from build123d import *

# Parameters (mm, degrees)
F1_DEPTH  = 495.3
F3_DEPTH  = 101.6
F4_R      = 63.5
F5_DEPTH  = 101.6
F7_DEPTH  = 127
F9_DEPTH  = 127
F11_DEPTH = 127
F13_DEPTH = 127


with BuildPart() as f1:
    # F0 (on Front) → F1 (new body)
    with BuildSketch(Plane.XZ):
        Polygon((635, -24.13), (635, 24.13), (-635, 24.13), (-635, 14.952256), (-635, -24.13), align=None)
        with BuildLine():
            Line((-635, -24.13), (-635, 14.952256))
            ThreePointArc((-635, 14.952256), (-763.72663, 119.691568), (-687.35112, 267.026731))
            Line((-687.35112, 267.026731), (-272.463288, 681.914564))
            Line((-272.463288, 681.914564), (-306.588261, 716.039537))
            Line((-306.588261, 716.039537), (-755.601067, 267.026731))
            ThreePointArc((-755.601067, 267.026731), (-792.572888, 81.156837), (-635, -24.13))
        make_face()
    extrude(amount=F1_DEPTH)

    # F2 (on face) → F3 (cut)
    with BuildSketch(Plane(origin=(-511.313899, 0, 511.313899), x_dir=(0, -1, 0), z_dir=(-0.707107, 0, 0.707107))):
        with BuildLine():
            ThreePointArc((152.4, 99.025774), (141.240768, 125.966543), (114.3, 137.125774))
            ThreePointArc((114.3, 137.125774), (87.359232, 72.085006), (152.4, 99.025774))
        make_face()
        with BuildLine():
            ThreePointArc((419.1, 99.025774), (407.940768, 125.966543), (381, 137.125774))
            ThreePointArc((381, 137.125774), (354.059232, 72.085006), (419.1, 99.025774))
        make_face()
    extrude(amount=-F3_DEPTH, mode=Mode.SUBTRACT)

    # F4 (on face) → F5 (cut)
    with BuildSketch(Plane.XY.offset(24.13)):
        with Locations((-177.8, -241.935)):
            Circle(F4_R)
        with BuildLine():
            Line((139.7, -247.65), (520.7, -247.65))
            ThreePointArc((520.7, -247.65), (502.101281, -202.748719), (457.2, -184.15))
            Line((457.2, -184.15), (203.2, -184.15))
            ThreePointArc((203.2, -184.15), (158.298719, -202.748719), (139.7, -247.65))
        make_face()
        with BuildLine():
            ThreePointArc((457.2, -311.15), (502.101281, -292.551281), (520.7, -247.65))
            Line((520.7, -247.65), (139.7, -247.65))
            ThreePointArc((139.7, -247.65), (158.298719, -292.551281), (203.2, -311.15))
            Line((203.2, -311.15), (457.2, -311.15))
        make_face()
    extrude(amount=-F5_DEPTH, mode=Mode.SUBTRACT)

    # F6 (on face) → F7 (cut)
    with BuildSketch(Plane(origin=(-511.313899, 0, 511.313899), x_dir=(0, -1, 0), z_dir=(-0.707107, 0, 0.707107))):
        with BuildLine():
            Line((127, 289.525774), (0, 289.525774))
            Line((0, 289.525774), (0, 162.525774))
            ThreePointArc((0, 162.525774), (37.197439, 252.328335), (127, 289.525774))
        make_face()
    extrude(amount=-F7_DEPTH, mode=Mode.SUBTRACT)

    # F8 (on face) → F9 (cut)
    with BuildSketch(Plane(origin=(-511.313899, 0, 511.313899), x_dir=(0, -1, 0), z_dir=(-0.707107, 0, 0.707107))):
        with BuildLine():
            Line((495.3, 162.525774), (495.3, 289.525774))
            Line((495.3, 289.525774), (368.3, 289.525774))
            ThreePointArc((368.3, 289.525774), (458.102561, 252.328335), (495.3, 162.525774))
        make_face()
    extrude(amount=-F9_DEPTH, mode=Mode.SUBTRACT)

    # F10 (on face) → F11 (cut)
    with BuildSketch(Plane(origin=(0, 0, -24.13), x_dir=(1, 0, 0), z_dir=(0, 0, -1))):
        with BuildLine():
            Line((635, 368.3), (635, 495.3))
            Line((635, 495.3), (508, 495.3))
            ThreePointArc((508, 495.3), (597.802561, 458.102561), (635, 368.3))
        make_face()
    extrude(amount=-F11_DEPTH, mode=Mode.SUBTRACT)

    # F12 (on face) → F13 (cut)
    with BuildSketch(Plane(origin=(0, 0, -24.13), x_dir=(1, 0, 0), z_dir=(0, 0, -1))):
        with BuildLine():
            Line((508, 0), (635, 0))
            Line((635, 0), (635, 127))
            ThreePointArc((635, 127), (597.802561, 37.197439), (508, 0))
        make_face()
    extrude(amount=-F13_DEPTH, mode=Mode.SUBTRACT)


solid = f1.part
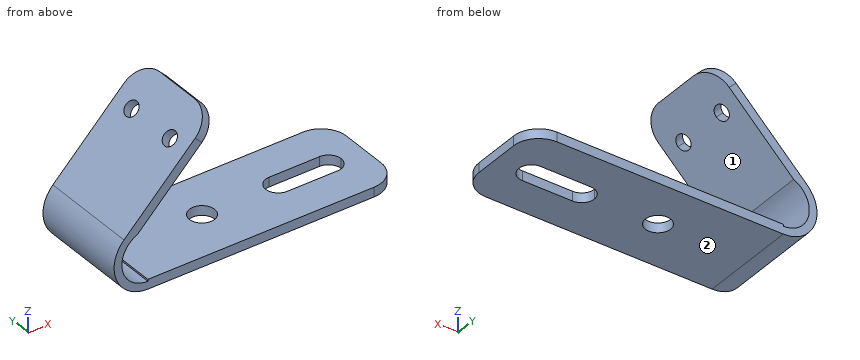
Design review of the part built by this model. Coordinates are the model's own, in mm. Face numbers are marked on the shaded views. A direction names the side the tool comes from. Round coordinates to 2 decimals unless told otherwise and drop trailing zeros. Write each loop counter-clockwise with the first axis right and the second up, starting at its lowest first coordinate (ties: lowest second). Pieces come first, ordered by that corner, then holes. Notation, with made-up numbers: (86.25, 73) -> (135.25, 73) arc R17 ccw to (135.25, 104) -> close; hole circle Ø4 at (-0.5, -37.75). An arc over 180 degrees is marked (long way). One line per question, with ' | ' between items.
(1) Insertion check: P1, Ø8, axis at y = -51, z = 162, coming from the -X side; P2, Ø1.5, axis at y = -52.5, z = 249, coming from the -X side; P3, Ø1, axis at y = -68.5, z = 147.5, coming from the +X side. Each pin has a flat end and moves straight along its axis. Give the tip position at first contact, or say it passes through.
Result sheet:
P1: x = -805.16 | P2: x = -771.82 | P3: x = -766.46
(2) Take a section at C-C, the plane z = 156. State the section outline as (x, y) points, and give its area (3 significant figures).
Result sheet:
outline: (-805.29, -495.3) -> (-766.12, -495.3) -> (-766.12, 0) -> (-805.29, 0) -> close | area: 19,400 mm2
(3) Wall thickness on line 1 (Y direction, x = -177.8, z = 4) (3 decimals); line 2 (Z direction, x = -48.5, y = -297); line 3 (Z direction, x = -279.5, y = -183.5): over which ranges is each line inside the solid? List them lowest first. Write a range as [from, to].
Result sheet:
line 1: [-495.3, -305.435], [-178.435, 0] | line 2: [-24.13, 24.13] | line 3: [-24.13, 24.13], [674.88, 688.95]
(4) Take a section at B-B, the plane x = -483. State the section outline as (y, z) points, and give its area (3 significant figures).
Result sheet:
outline: (-495.3, -24.13) -> (0, -24.13) -> (0, 24.13) -> (-495.3, 24.13) -> close; (-495.3, 471.38) -> (0, 471.38) -> (0, 539.63) -> (-495.3, 539.63) -> close | area: 57,700 mm2
(5) Take a section at A-A, the plane x = -177.8. State the section outline as (y, z) points (3 decimals), and give its area (3 significant figures).
Result sheet:
outline: (-495.3, -24.13) -> (-305.435, -24.13) -> (-305.435, 24.13) -> (-495.3, 24.13) -> close; (-178.435, -24.13) -> (0, -24.13) -> (0, 24.13) -> (-178.435, 24.13) -> close | area: 17,800 mm2
(6) Machinability: for the marked faces 1 and 2, which of the approach directions +Z, -Z, +X, -X, +Y, -Y give a long, thin tool a straight path to every point of the face, cutting with its end or side? Answer none if there is none.
Result sheet:
face 1: +X, +Y, -Y | face 2: -Z, +X, -X, +Y, -Y
(7) Take a section at D-D, the plane z = 417.5. State the section outline as (x, y) points, and give its area (3 significant figures).
Result sheet:
outline: (-605.13, -495.3) -> (-536.88, -495.3) -> (-536.88, 0) -> (-605.13, 0) -> close | area: 33,800 mm2
